For this review, take the finished solid that the model builds, in its own axes (mm). A direction names the side the tool comes from. Give positions to 0.01 mm unless a question says otherwise; leave off trailing zeros. Order: outer loops, then holes, each group sorted by start corner. A loop starts at its lowest first (then second) coordinate and runs counter-clockwise, first axis right, second up. Notation, with made-up numbers: M 74.5,45 L 119.5,45 A15 ccw 119.5,74 Z; hole C -7,77.5 d9. An arc over 180 degrees is marked long. Use CSV: the item, a comma, the result in double quotes. Start each with the question number.
(1) Clearance check with flat-ended pins moving along their axes: P1, Ø4, axis at y = 2.5, z = -16, coming from the -X side; P2, Ø19, axis at x = -17, y = 16.5, coming from the -Z side; P3, Ø2, axis at x = -34, z = -20, coming from the +Y side; P4, Ø4, axis at y = 1, z = -10.5, coming from the +X side. State where each tip first meets the part, or that it passes through.
(2) Wall thickness on L1, parallel to Z at x = 17.5, y = 16; L2, parallel to Y at x = -19, z = -7; L3, parallel to Z at x = 35.5, y = -3: over which ranges is each line inside the solid? List them lowest first. Write a range as from..to.
(3) Tool access review of faces 1 (the face through (-1, 0, -8)), 2 (the face through (70, 14, 21)): name each direction out of +Z, -Z, +X, -X, +Y, -Y from which nothing blocks a thin tool from reaching the whole face with its end or side.
(4) Consider section A-A (y = 9.5). Write out the cut boundary in (x, z).
(5) Consider section D-D (x = -55.5). Write out the cut boundary in (y, z), and give its area (3 significant figures).
(6) Consider section B-B (x = -1). Write out the cut boundary in (y, z), and give its area (3 significant figures).
(7) Consider section C-C (z = 10.5). Write out the cut boundary in (x, y), and give its area (3 significant figures).
```python
from build123d import *

# Parameters (mm, degrees)
SKETCH1_W                    = 140
SKETCH1_H                    = 50
BASE_FLANGE1_DEPTH           = 8
EDGE_FLANGE1_STRIP_W         = 48
EDGE_FLANGE1_STRIP_H         = 8
EDGE_FLANGE1_STRIP_CUT_DEPTH = 140
EDGE_FLANGE1_DEPTH           = 140
CHAMFER1_SIZE                = 43
CHAMFER1_SIZE2               = 30.108924143
MIRROR2_START                = 47.016267246
MIRROR2_OUTLINE_W            = 55
MIRROR2_OUTLINE_H            = 41
MIRROR2_DEPTH                = 24.663786763


# Read off the part's stored shape, not the designer's step: Mirror2
# Sheet-metal steps are written as plain solids
with BuildPart() as part:
    # Sketch1 → Base-Flange1 (new body)
    with BuildSketch(Plane(origin=(0, 0, 0), x_dir=(1, 0, 0), z_dir=(0, 1, 0))):
        Rectangle(SKETCH1_W, SKETCH1_H)
    extrude(amount=-BASE_FLANGE1_DEPTH)

    # Edge-Flange1 strip (across the edge) → Edge-Flange1 strip cut (cut)
    with BuildSketch(Plane(origin=(-70, 0, 25), x_dir=(0, 0, -1), z_dir=(1, 0, 0))):
        with Locations((-8, -4)):
            Rectangle(EDGE_FLANGE1_STRIP_W, EDGE_FLANGE1_STRIP_H)
    extrude(amount=EDGE_FLANGE1_STRIP_CUT_DEPTH, mode=Mode.SUBTRACT)

    # Edge-Flange1 section (across the edge) → Edge-Flange1 (add)
    with BuildSketch(Plane(origin=(-70, 0, 25), x_dir=(0, 0, -1), z_dir=(1, 0, 0))):
        with BuildLine():
            Line((0, 8), (0, 32))
            Line((0, 32), (8, 32))
            Line((8, 32), (8, 8))
            ThreePointArc((8, 8), (10.343145751, 2.343145751), (16, 0))
            Line((16, 0), (16, -8))
            ThreePointArc((16, -8), (4.686291501, -3.313708499), (0, 8))
        make_face()
    extrude(amount=EDGE_FLANGE1_DEPTH)

    # Chamfer1
    chamfer1_edges = [part.edges().sort_by_distance(p)[0] for p in [
        (-70, -4, -25),
    ]]
    chamfer1_side = [part.faces().sort_by_distance(p)[0] for p in [
        (-70, -0.640312424, -8),
    ]]
    chamfer(chamfer1_edges, length=CHAMFER1_SIZE, length2=CHAMFER1_SIZE2, reference=chamfer1_side[0])

    # Mirror2 outline → Mirror2 (cut)
    with BuildSketch(Plane(origin=(0, 0, 0), x_dir=(0.5735764363510512, 0, 0.8191520442889882), z_dir=(0.8191520442889882, 0, -0.5735764363510512)).offset(MIRROR2_START)):
        with Locations((28.5, -12.5)):
            Rectangle(MIRROR2_OUTLINE_W, MIRROR2_OUTLINE_H)
    extrude(amount=MIRROR2_DEPTH, mode=Mode.SUBTRACT)


solid = part.part
```
Check result:
1,P1,"passes through"
1,P2,"stops at z = 16.94"
1,P3,"stops at y = 0"
1,P4,"stops at x = 51.26"
2,L1,"z = 17..25"
2,L2,"y = -8..0"
2,L3,"z = -25..20.62"
3,face 1,"-Z, +X, -X, +Y"
3,face 2,"+Z, -Z, +X, +Y, -Y"
4,outline,"M -70,18 L -69.3,17 L 69.3,17 L 70,18 L 70,25 L -70,25 Z"
5,outline,"M -8,-2.71 L 0,-2.71 L 0,9 A8 cw 8,17 L 32,17 L 32,25 L 8,25 A16 ccw -8,9 Z"
5,area,"436 mm^2"
6,outline,"M -8,-25 L 0,-25 L 0,9 A8 cw 8,17 L 32,17 L 32,25 L 8,25 A16 ccw -8,9 Z"
6,area,"615 mm^2"
7,outline,"M -64.75,-7.93 L 64.75,-7.93 L 64.75,0.14 L -64.75,0.14 Z"
7,area,"1,050 mm^2"
